```python
from build123d import *

# Parameters (mm, degrees)
BOSS_EXTRUDE2_DEPTH = 2.5


with BuildPart() as part:
    # Sketch1 → Boss-Extrude2 (new body)
    with BuildSketch(Plane(origin=(0, 0, 0), x_dir=(1, 0, 0), z_dir=(0, 1, 0))):
        with BuildLine():
            Line((-52.5, 32.5), (-41.25, 32.5))
            Line((-41.25, 32.5), (-41.25, 35))
            Line((-41.25, 35), (-11.25, 35))
            Line((-11.25, 35), (-11.25, 32.5))
            Line((-11.25, 32.5), (11.25, 32.5))
            Line((11.25, 32.5), (11.25, 35))
            Line((11.25, 35), (41.25, 35))
            Line((41.25, 35), (41.25, 32.5))
            Line((41.25, 32.5), (52.5, 32.5))
            ThreePointArc((52.5, 32.5), (66.642135624, 26.642135624), (72.5, 12.5))
            Line((72.5, 12.5), (72.5, -12.5))
            ThreePointArc((72.5, -12.5), (66.642135624, -26.642135624), (52.5, -32.5))
            Line((52.5, -32.5), (41.25, -32.5))
            Line((41.25, -32.5), (41.25, -35))
            Line((41.25, -35), (11.25, -35))
            Line((11.25, -35), (11.25, -32.5))
            Line((11.25, -32.5), (-11.25, -32.5))
            Line((-11.25, -32.5), (-11.25, -35))
            Line((-11.25, -35), (-41.25, -35))
            Line((-41.25, -35), (-41.25, -32.5))
            Line((-41.25, -32.5), (-52.5, -32.5))
            ThreePointArc((-52.5, -32.5), (-66.642135624, -26.642135624), (-72.5, -12.5))
            Line((-72.5, -12.5), (-72.5, 12.5))
            ThreePointArc((-72.5, 12.5), (-66.642135624, 26.642135624), (-52.5, 32.5))
        make_face()
    extrude(amount=BOSS_EXTRUDE2_DEPTH)


solid = part.part
```
Geometry: final body of the model. Coordinates: model frame, mm. A direction names the side the tool comes from. Coordinates: 2 decimals unless noted, no trailing zeros. Order: outer loops, then holes, each group sorted by start corner. A loop starts at its lowest first (then second) coordinate and runs counter-clockwise, first axis right, second up. Notation, with made-up numbers: (13.5, 72.5) - (55.5, 72.5) arc R10 cw to (55.5, 84.5) - close; hole circle Ø8 at (33, 35.5). An arc over 180 degrees is marked (long way). Return JSON: item names as keys, results as strings. Group by question number.
1. Cut plane C-C (x = 59.5). Output: boundary loops of the cut face in (y, z) (3 decimals).
2. Pull-direction query (X, two-part tool) for faces 4 (the face through (47, 1, -32.5)), 5 (the face through (-11.25, 1, 34)), 6 (the face through (72.5, 1, 0)); classes: pulls with the +X half, pulls with the -X half, needs draft (parallel to the pull), parting line crosses it, or undercut.
3. Cut plane A-A (y = 1.1). Output: boundary loops of the cut face in (x, z).
4. Cut plane B-B (z = 28.5). Output: boundary loops of the cut face in (x, y), plus the area to 4 significant figures.
5. Set-up query: faces 1 (the face through (47, 1, 32.5)), 2 (the face through (-47, 1, -32.5)), 3 (the face through (0, 1, 32.5)). Return all of +Z, -Z, +X, -X, +Y, -Y with unobstructed straight access to the full face (end or side cutting, diameter ignored); none if empty.
6. Pin query (flat end, axial travel): pin 1 (0.8 mm diameter, centred on y = 1, z = -33.5, fed in from +X); pin 2 (1.5 mm diameter, centred on x = 54.5, y = 0.5, fed in from -Z); pin 3 (0.8 mm diameter, centred on y = 1.5, z = -33, fed in from -X). Return the tip coordinate at first contact, or that it passes through.
7. Material intervals for line 1 along X through (y, z) = (1.1, -13); line 2 along Z through (x, y) = (44, 1.9); line 3 along X through (y, z) = (0.25, 30), sorted ascending. Write a range as [from, to].
Resolved:
{
 "1": {"outline": "(0, -31.235) - (2.5, -31.235) - (2.5, 31.235) - (0, 31.235) - close"},
 "2": {"face 4": "needs draft", "face 5": "undercut", "face 6": "pulls with the +X half"},
 "3": {"outline": "(-72.5, -12.5) arc R20 ccw to (-52.5, -32.5) - (-41.25, -32.5) - (-41.25, -35) - (-11.25, -35) - (-11.25, -32.5) - (11.25, -32.5) - (11.25, -35) - (41.25, -35) - (41.25, -32.5) - (52.5, -32.5) arc R20 ccw to (72.5, -12.5) - (72.5, 12.5) arc R20 ccw to (52.5, 32.5) - (41.25, 32.5) - (41.25, 35) - (11.25, 35) - (11.25, 32.5) - (-11.25, 32.5) - (-11.25, 35) - (-41.25, 35) - (-41.25, 32.5) - (-52.5, 32.5) arc R20 ccw to (-72.5, 12.5) - close"},
 "4": {"outline": "(-64.5, 0) - (64.5, 0) - (64.5, 2.5) - (-64.5, 2.5) - close", "area": "322.5 mm²"},
 "5": {"face 1": "+Z, +X, +Y, -Y", "face 2": "-Z, -X, +Y, -Y", "face 3": "+Z, +Y, -Y"},
 "6": {"pin 1": "stops at x = 41.25", "pin 2": "stops at z = -32.46", "pin 3": "stops at x = -41.25"},
 "7": {"line 1": "x = [-72.49, 72.49]", "line 2": "z = [-32.5, 32.5]", "line 3": "x = [-62.18, 62.18]"}
}
